For this review, take the finished solid that the model builds, in its own axes (mm). Face numbers are marked on the shaded views. A direction names the side the tool comes from. Give positions to 0.01 mm unless a question says otherwise; leave off trailing zeros. Write each loop counter-clockwise with the first axis right and the second up, starting at its lowest first coordinate (ties: lowest second). Pieces come first, ordered by that corner, then holes.
1) We need section C-C on y = 31.5. Give the boundary of the cut face in (x, z).
2) Machinability: for the marked faces 1 and 2, which of the approach directions +Z, -Z, +X, -X, +Y, -Y give a long, thin tool a straight path to every point of the face, cutting with its end or side? Answer none if there is none.
3) For P1, Ø4.5, axis at x = 30, z = 144, coming from the +Y side; P2, Ø3.5, axis at x = -79, z = 87, coming from the -Y side; P3, Ø5, axis at x = 4, z = 196, coming from the +Y side; P4, Ø2.5, axis at x = 13.911, z = 139.416, coming from the +Y side, all flat-tipped, find the tip position at first contact; note any pin that passes through.
4) We need section B-B on x = -112.5. Give the boundary of the cut face in (y, z).
5) Wall thickness on line 1 along Z through (x, y) = (30, 6); line 2 along Z through (x, y) = (30, 3.65); line 3 along X through (y, z) = (1, 144): over which ranges is each line inside the solid? List them lowest first.
6) We need section A-A on z = 118. Give the boundary of the cut face in (x, y), and give its area (3 significant figures).
7) Draft analysis for pull direction Z (two halves, no side actions). For the marked faces 3, 4 and 5, state which applies: pulls with the +Z half, pulls with the -Z half, needs draft (parallel to the pull), parting line crosses it, or undercut.
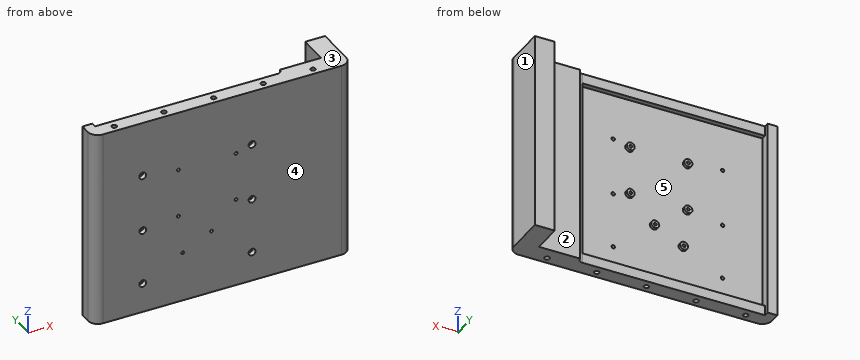
from build123d import *

# Parameters (mm, degrees)
EXTRUDE_1_DEPTH     = 200
CUT_EXTRUDE_1_REACH = 245.721
CUT_EXTRUDE_2_REACH = 243.091
SKETCH_4_R          = 1.75
SKETCH_4_R_2        = 1.5
SKETCH_6_W          = 183.452994616
SKETCH_6_H          = 180
CUT_EXTRUDE_4_DEPTH = 5
EXTRUDE_START       = 3
SKETCH_7_R          = 4
SKETCH_7_R_2        = 1.5
EXTRUDE_2_DEPTH     = 3
SKETCH_8_R          = 2.5
CUT_EXTRUDE_5_DEPTH = 15
SKETCH_9_R          = 3.5
CUT_EXTRUDE_6_DEPTH = 5


with BuildPart() as part:
    # 草图1 → 凸台-拉伸1 (new body)
    with BuildSketch(Plane.XY):
        with BuildLine():
            Line((-120, 0), (120, 0))
            ThreePointArc((120, 0), (127.071067812, 2.928932188), (130, 10))
            Line((130, 10), (130, 49.985304377))
            Line((130, 49.985304377), (130, 50))
            Line((130, 50), (110, 50))
            Line((110, 50), (110, 48.038475773))
            Line((110, 48.038475773), (110, 20))
            Line((110, 20), (-110, 20))
            Line((-110, 20), (-130, 20))
            Line((-130, 20), (-130, 10))
            ThreePointArc((-130, 10), (-127.071067812, 2.928932188), (-120, 0))
        make_face()
    extrude(amount=EXTRUDE_1_DEPTH)

    # 草图3 → 切除-拉伸1 (cut, up to next)
    with BuildSketch(Plane.XY.offset(200), mode=Mode.PRIVATE) as cut_extrude_1_sk1:
        with BuildLine():
            Line((-120, 20), (68.452994616, 20))
            ThreePointArc((68.452994616, 20), (66.988528522, 16.464466094), (63.452994616, 15))
            Line((63.452994616, 15), (-120, 15))
            Line((-120, 15), (-120, 20))
        make_face()
    cut_extrude_1_tool1 = extrude(cut_extrude_1_sk1.sketch, amount=-CUT_EXTRUDE_1_REACH, mode=Mode.PRIVATE) & part.part
    add(cut_extrude_1_tool1.solids().sort_by_distance((-26.306684, 17.507921, 200))[0], mode=Mode.SUBTRACT)

    # 草图4 → 切除-拉伸2 (cut, up to next)
    with BuildSketch(Plane(origin=(0, 15, 0), x_dir=(1, 0, 0), z_dir=(0, 1, 0)), mode=Mode.PRIVATE) as cut_extrude_2_sk1:
        with Locations(Location((30, -30, 0), (0, 0, 180))):
            Circle(SKETCH_4_R)
    cut_extrude_2_tool1 = extrude(cut_extrude_2_sk1.sketch, amount=-CUT_EXTRUDE_2_REACH, mode=Mode.PRIVATE) & part.part
    # 草图4 → 切除-拉伸2 (cut, up to next)
    with BuildSketch(Plane(origin=(0, 15, 0), x_dir=(1, 0, 0), z_dir=(0, 1, 0)), mode=Mode.PRIVATE) as cut_extrude_2_sk2:
        with Locations(Location((30, -86, 0), (0, 0, 180))):
            Circle(SKETCH_4_R)
    cut_extrude_2_tool2 = extrude(cut_extrude_2_sk2.sketch, amount=-CUT_EXTRUDE_2_REACH, mode=Mode.PRIVATE) & part.part
    # 草图4 → 切除-拉伸2 (cut, up to next)
    with BuildSketch(Plane(origin=(0, 15, 0), x_dir=(1, 0, 0), z_dir=(0, 1, 0)), mode=Mode.PRIVATE) as cut_extrude_2_sk3:
        with Locations(Location((30, -144, 0), (0, 0, 180))):
            Circle(SKETCH_4_R)
    cut_extrude_2_tool3 = extrude(cut_extrude_2_sk3.sketch, amount=-CUT_EXTRUDE_2_REACH, mode=Mode.PRIVATE) & part.part
    # 草图4 → 切除-拉伸2 (cut, up to next)
    with BuildSketch(Plane(origin=(0, 15, 0), x_dir=(1, 0, 0), z_dir=(0, 1, 0)), mode=Mode.PRIVATE) as cut_extrude_2_sk4:
        with Locations(Location((-80, -144, 0), (0, 0, 180))):
            Circle(SKETCH_4_R)
    cut_extrude_2_tool4 = extrude(cut_extrude_2_sk4.sketch, amount=-CUT_EXTRUDE_2_REACH, mode=Mode.PRIVATE) & part.part
    # 草图4 → 切除-拉伸2 (cut, up to next)
    with BuildSketch(Plane(origin=(0, 15, 0), x_dir=(1, 0, 0), z_dir=(0, 1, 0)), mode=Mode.PRIVATE) as cut_extrude_2_sk5:
        with Locations(Location((-80, -86, 0), (0, 0, 180))):
            Circle(SKETCH_4_R)
    cut_extrude_2_tool5 = extrude(cut_extrude_2_sk5.sketch, amount=-CUT_EXTRUDE_2_REACH, mode=Mode.PRIVATE) & part.part
    # 草图4 → 切除-拉伸2 (cut, up to next)
    with BuildSketch(Plane(origin=(0, 15, 0), x_dir=(1, 0, 0), z_dir=(0, 1, 0)), mode=Mode.PRIVATE) as cut_extrude_2_sk6:
        with Locations(Location((-80, -30, 0), (0, 0, 180))):
            Circle(SKETCH_4_R)
    cut_extrude_2_tool6 = extrude(cut_extrude_2_sk6.sketch, amount=-CUT_EXTRUDE_2_REACH, mode=Mode.PRIVATE) & part.part
    # 草图4 → 切除-拉伸2 (cut, up to next)
    with BuildSketch(Plane(origin=(0, 15, 0), x_dir=(1, 0, 0), z_dir=(0, 1, 0)), mode=Mode.PRIVATE) as cut_extrude_2_sk7:
        with Locations(Location((-10.76, -64.486, 0), (0, 0, 180))):
            Circle(SKETCH_4_R_2)
    cut_extrude_2_tool7 = extrude(cut_extrude_2_sk7.sketch, amount=-CUT_EXTRUDE_2_REACH, mode=Mode.PRIVATE) & part.part
    # 草图4 → 切除-拉伸2 (cut, up to next)
    with BuildSketch(Plane(origin=(0, 15, 0), x_dir=(1, 0, 0), z_dir=(0, 1, 0)), mode=Mode.PRIVATE) as cut_extrude_2_sk8:
        with Locations(Location((-39.76, -50.486, 0), (0, 0, 180))):
            Circle(SKETCH_4_R_2)
    cut_extrude_2_tool8 = extrude(cut_extrude_2_sk8.sketch, amount=-CUT_EXTRUDE_2_REACH, mode=Mode.PRIVATE) & part.part
    # 草图4 → 切除-拉伸2 (cut, up to next)
    with BuildSketch(Plane(origin=(0, 15, 0), x_dir=(1, 0, 0), z_dir=(0, 1, 0)), mode=Mode.PRIVATE) as cut_extrude_2_sk9:
        with Locations(Location((-44.089, -90.416, 0), (0, 0, 180))):
            Circle(SKETCH_4_R_2)
    cut_extrude_2_tool9 = extrude(cut_extrude_2_sk9.sketch, amount=-CUT_EXTRUDE_2_REACH, mode=Mode.PRIVATE) & part.part
    # 草图4 → 切除-拉伸2 (cut, up to next)
    with BuildSketch(Plane(origin=(0, 15, 0), x_dir=(1, 0, 0), z_dir=(0, 1, 0)), mode=Mode.PRIVATE) as cut_extrude_2_sk10:
        with Locations(Location((13.911, -90.416, 0), (0, 0, 180))):
            Circle(SKETCH_4_R_2)
    cut_extrude_2_tool10 = extrude(cut_extrude_2_sk10.sketch, amount=-CUT_EXTRUDE_2_REACH, mode=Mode.PRIVATE) & part.part
    # 草图4 → 切除-拉伸2 (cut, up to next)
    with BuildSketch(Plane(origin=(0, 15, 0), x_dir=(1, 0, 0), z_dir=(0, 1, 0)), mode=Mode.PRIVATE) as cut_extrude_2_sk11:
        with Locations(Location((13.911, -139.416, 0), (0, 0, 180))):
            Circle(SKETCH_4_R_2)
    cut_extrude_2_tool11 = extrude(cut_extrude_2_sk11.sketch, amount=-CUT_EXTRUDE_2_REACH, mode=Mode.PRIVATE) & part.part
    # 草图4 → 切除-拉伸2 (cut, up to next)
    with BuildSketch(Plane(origin=(0, 15, 0), x_dir=(1, 0, 0), z_dir=(0, 1, 0)), mode=Mode.PRIVATE) as cut_extrude_2_sk12:
        with Locations(Location((-44.089, -139.416, 0), (0, 0, 180))):
            Circle(SKETCH_4_R_2)
    cut_extrude_2_tool12 = extrude(cut_extrude_2_sk12.sketch, amount=-CUT_EXTRUDE_2_REACH, mode=Mode.PRIVATE) & part.part
    add(cut_extrude_2_tool1.solids().sort_by_distance((30, 15, 30))[0], mode=Mode.SUBTRACT)
    add(cut_extrude_2_tool2.solids().sort_by_distance((30, 15, 86))[0], mode=Mode.SUBTRACT)
    add(cut_extrude_2_tool3.solids().sort_by_distance((30, 15, 144))[0], mode=Mode.SUBTRACT)
    add(cut_extrude_2_tool4.solids().sort_by_distance((-80, 15, 144))[0], mode=Mode.SUBTRACT)
    add(cut_extrude_2_tool5.solids().sort_by_distance((-80, 15, 86))[0], mode=Mode.SUBTRACT)
    add(cut_extrude_2_tool6.solids().sort_by_distance((-80, 15, 30))[0], mode=Mode.SUBTRACT)
    add(cut_extrude_2_tool7.solids().sort_by_distance((-10.76, 15, 64.486))[0], mode=Mode.SUBTRACT)
    add(cut_extrude_2_tool8.solids().sort_by_distance((-39.76, 15, 50.486))[0], mode=Mode.SUBTRACT)
    add(cut_extrude_2_tool9.solids().sort_by_distance((-44.089, 15, 90.416))[0], mode=Mode.SUBTRACT)
    add(cut_extrude_2_tool10.solids().sort_by_distance((13.911, 15, 90.416))[0], mode=Mode.SUBTRACT)
    add(cut_extrude_2_tool11.solids().sort_by_distance((13.911, 15, 139.416))[0], mode=Mode.SUBTRACT)
    add(cut_extrude_2_tool12.solids().sort_by_distance((-44.089, 15, 139.416))[0], mode=Mode.SUBTRACT)

    # 草图6 → 切除-拉伸4 (cut)
    with BuildSketch(Plane(origin=(0, 15, 0), x_dir=(1, 0, 0), z_dir=(0, 1, 0))):
        with Locations((-28.273502692, -100)):
            Rectangle(SKETCH_6_W, SKETCH_6_H)
    extrude(amount=-CUT_EXTRUDE_4_DEPTH, mode=Mode.SUBTRACT)

    # 草图7 → 凸台-拉伸2 (add)
    # profile 1 of 6: a face of its own
    with BuildSketch(Plane(origin=(0, 10, 0), x_dir=(1, 0, 0), z_dir=(0, 1, 0)).offset(EXTRUDE_START)):
        with Locations(Location((-39.76, -50.486, 0), (0, 0, 180))):
            Circle(SKETCH_7_R)
        with Locations(Location((-39.76, -50.486, 0), (0, 0, 180))):
            Circle(SKETCH_7_R_2, mode=Mode.SUBTRACT)
    # profile 2 of 6: a face of its own
    with BuildSketch(Plane(origin=(0, 10, 0), x_dir=(1, 0, 0), z_dir=(0, 1, 0)).offset(EXTRUDE_START)):
        with Locations(Location((-10.76, -64.486, 0), (0, 0, 180))):
            Circle(SKETCH_7_R)
        with Locations(Location((-10.76, -64.486, 0), (0, 0, 180))):
            Circle(SKETCH_7_R_2, mode=Mode.SUBTRACT)
    # profile 3 of 6: a face of its own
    with BuildSketch(Plane(origin=(0, 10, 0), x_dir=(1, 0, 0), z_dir=(0, 1, 0)).offset(EXTRUDE_START)):
        with Locations(Location((13.911, -90.416, 0), (0, 0, 180))):
            Circle(SKETCH_7_R)
        with Locations(Location((13.911, -90.416, 0), (0, 0, 180))):
            Circle(SKETCH_7_R_2, mode=Mode.SUBTRACT)
    # profile 4 of 6: a face of its own
    with BuildSketch(Plane(origin=(0, 10, 0), x_dir=(1, 0, 0), z_dir=(0, 1, 0)).offset(EXTRUDE_START)):
        with Locations(Location((13.911, -139.416, 0), (0, 0, 180))):
            Circle(SKETCH_7_R)
        with Locations(Location((13.911, -139.416, 0), (0, 0, 180))):
            Circle(SKETCH_7_R_2, mode=Mode.SUBTRACT)
    # profile 5 of 6: a face of its own
    with BuildSketch(Plane(origin=(0, 10, 0), x_dir=(1, 0, 0), z_dir=(0, 1, 0)).offset(EXTRUDE_START)):
        with Locations(Location((-44.089, -139.416, 0), (0, 0, 180))):
            Circle(SKETCH_7_R)
        with Locations(Location((-44.089, -139.416, 0), (0, 0, 180))):
            Circle(SKETCH_7_R_2, mode=Mode.SUBTRACT)
    # profile 6 of 6: a face of its own
    with BuildSketch(Plane(origin=(0, 10, 0), x_dir=(1, 0, 0), z_dir=(0, 1, 0)).offset(EXTRUDE_START)):
        with Locations(Location((-44.089, -90.416, 0), (0, 0, 180))):
            Circle(SKETCH_7_R)
        with Locations(Location((-44.089, -90.416, 0), (0, 0, 180))):
            Circle(SKETCH_7_R_2, mode=Mode.SUBTRACT)
    extrude(amount=-EXTRUDE_2_DEPTH)

    # 草图8 → 切除-拉伸5 (cut)
    with BuildSketch(Plane(origin=(0, 0, 0), x_dir=(-1, 0, 0), z_dir=(0, 0, -1))):
        with Locations((105, 7)):
            Circle(SKETCH_8_R)
        with Locations((55, 7)):
            Circle(SKETCH_8_R)
        with Locations((5, 7)):
            Circle(SKETCH_8_R)
        with Locations((-45, 7)):
            Circle(SKETCH_8_R)
        with Locations((-95, 7)):
            Circle(SKETCH_8_R)
    cut_extrude_5 = extrude(amount=-CUT_EXTRUDE_5_DEPTH, mode=Mode.SUBTRACT)

    # 镜向1: 切除-拉伸5 across plane
    add(cut_extrude_5.mirror(Plane(origin=(0, 0, 100), x_dir=(1, 0, 0), z_dir=(0, 0, -1))), mode=Mode.SUBTRACT)

    # 草图9 → 切除-拉伸6 (cut)
    with BuildSketch(Plane.XZ):
        with Locations((-80, 144)):
            Circle(SKETCH_9_R)
        with Locations((30, 144)):
            Circle(SKETCH_9_R)
        with Locations((30, 86)):
            Circle(SKETCH_9_R)
        with Locations((30, 30)):
            Circle(SKETCH_9_R)
        with Locations((-80, 30)):
            Circle(SKETCH_9_R)
        with Locations((-80, 86)):
            Circle(SKETCH_9_R)
    extrude(amount=-CUT_EXTRUDE_6_DEPTH, mode=Mode.SUBTRACT)


solid = part.part
Results list:
1. outline: (110, 0) - (130, 0) - (130, 200) - (110, 200) - close
2. face 1: +Z, -Z, +X, +Y, -Y
2. face 2: +Z, -Z, -X, +Y
3. P1: stops at y = 10
3. P2: stops at y = 5
3. P3: stops at y = 15
3. P4: passes through
4. outline: (0, 0) - (15, 0) - (15, 10) - (10, 10) - (10, 190) - (15, 190) - (15, 200) - (0, 200) - close
5. line 1: z = 0 to 28.25, 31.75 to 84.25, 87.75 to 142.25, 145.75 to 200
5. line 2: z = 0 to 26.5, 33.5 to 82.5, 89.5 to 140.5, 147.5 to 200
5. line 3: x = -124.36 to -83.5, -76.5 to 26.5, 33.5 to 124.36
6. outline: (-130, 10) arc R10 ccw to (-120, 0) - (120, 0) arc R10 ccw to (130, 10) - (130, 50) - (110, 50) - (110, 20) - (68.45, 20) arc R5 cw to (63.45, 15) - (63.45, 10) - (-120, 10) - (-120, 20) - (-130, 20) - close
6. area: 3,900 mm2
7. face 3: pulls with the +Z half
7. face 4: needs draft
7. face 5: undercut
